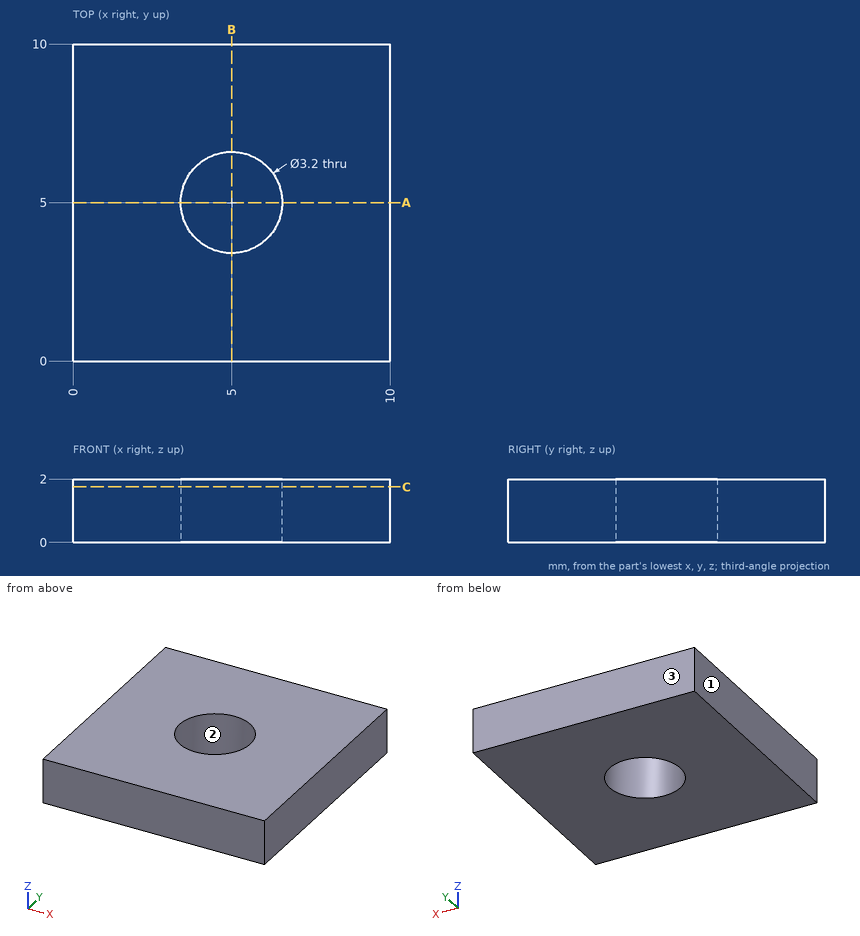
Here's the drawing with two shaded views (mm, measured from the low corner). I have some questions. Coordinates: 2 decimals unless noted, no trailing zeros. Loops run counter-clockwise (first coordinate to the right, second up) from the corner with the lowest first, then second, coordinate; pieces in that order, holes last. Notation, with made-up numbers: (25.5, 13) -> (81.5, 13) arc R15 ccw to (81.5, 34) -> close; hole circle Ø8 at (-4, 43.5). An arc over 180 degrees is marked (long way). Use one line per item in the form item = value. Start each with the question number.
(1) Will this pin go through, and if not, where does the flat tip stop? pin 1 (5 mm diameter, centred on x = 5, y = 5, fed in from +Z).
(2) We'd pull the mould along Y, two halves only. Please class the marked faces 1, 2 and 3: pulls with the +Y half, pulls with the -Y half, needs draft (parallel to the pull), parting line crosses it, or undercut.
(3) If we section it at C-C (z = 1.75): Please give me the cut outline in (x, y).
(4) Please list where these lines run through material, in increasing order: line 1 along Y through (x, z) = (5, 1.4); line 2 along Y through (x, z) = (4, 1.25).
(5) If we section it at A-A (y = 5): Please give me the cut outline in (x, z), then the cut area to 3 significant figures.
Verdict:
q1.pin_1 = 2
q2.face_1 = needs draft
q2.face_2 = undercut
q2.face_3 = pulls with the +Y half
q3.outline = (0, 0) -> (10, 0) -> (10, 10) -> (0, 10) -> close; hole circle Ø3.2 at (5, 5)
q4.line_1 = 0 to 3.4, 6.6 to 10
q4.line_2 = 0 to 3.75, 6.25 to 10
q5.outline = (0, 0) -> (3.4, 0) -> (3.4, 2) -> (0, 2) -> close; (6.6, 0) -> (10, 0) -> (10, 2) -> (6.6, 2) -> close
q5.area = 13.6 mm²
